Part print with two shaded views. Sizes in mm from the minimum x, y, z corner. A direction names the side the tool comes from. Give positions to 0.01 mm unless a question says otherwise; leave off trailing zeros. Order: outer loops, then holes, each group sorted by start corner. A loop starts at its lowest first (then second) coordinate and runs counter-clockwise, first axis right, second up.
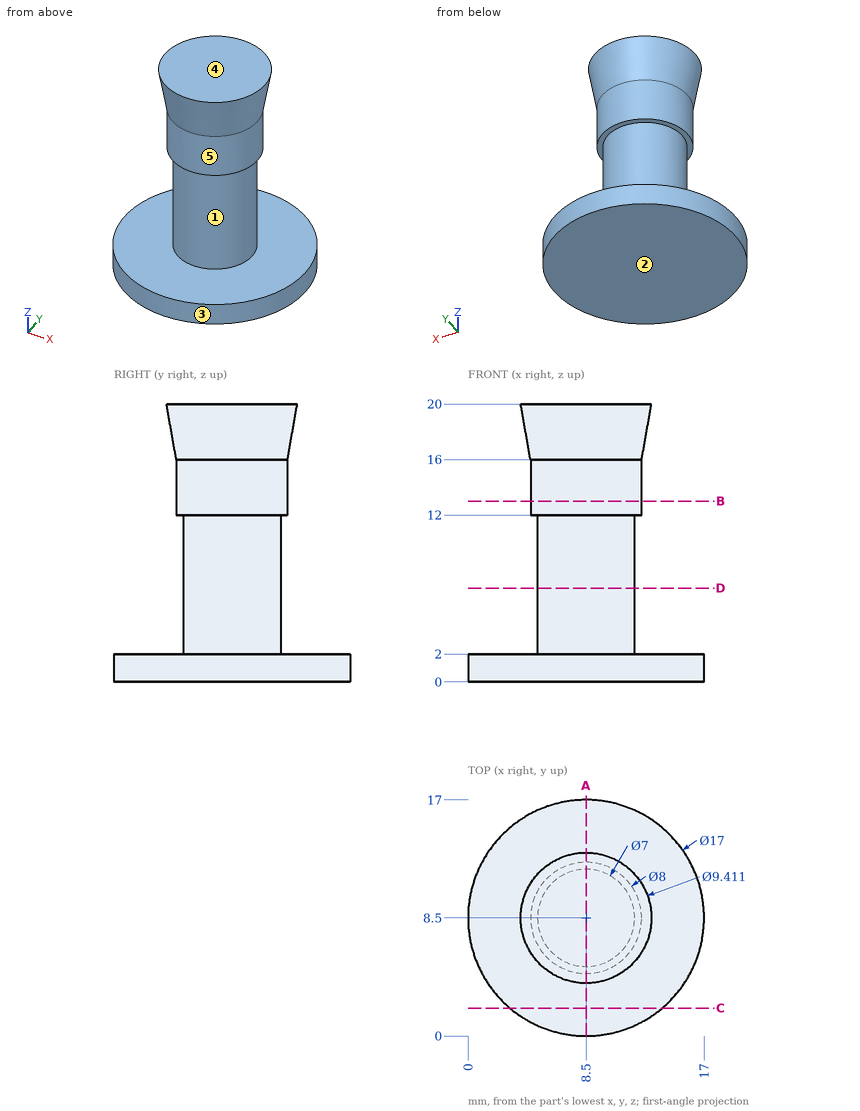
Item 1: Slice it at C-C (y = 2). Give the cut face in (x, z), and give its area (3 significant figures).
Item 2: Two-plate mould, pull along Z, no slides. Class the marked faces 1, 2 and 3: released by +Z, released by -Z, zero draft, split by the parting line, or undercut.
Item 3: Slice it at A-A (x = 8.5). Give the cut face in (y, z) (1 decimal), and give its area (3 significant figures).
Item 4: Tool access for the marked faces 4 and 5: list every direction of +Z, -Z, +X, -X, +Y, -Y with a clear straight run to the whole face (end or side of a thin tool).
Item 5: Drop flat-ended pins along their axis: pin 1 Ø6 at (x, z) = (7, 7.5) entering from -Y; pin 2 Ø8 at (y, z) = (12, 6.5) entering from -X; pin 3 Ø1.5 at (y, z) = (10.5, 14) entering from -X. Give the stop position or say it passes through.
Item 6: Wall check: L1, parallel to Z at x = 15.25, y = 4; L2, parallel to X at y = 7.5, z = 1.75; L3, parallel to X at y = 6, z = 14. Give the ranges that are in metal, low to high.
Item 7: Slice it at D-D (z = 6.75). Give the cut face in (x, y).
Item 8: Slice it at B-B (z = 13). Give the cut face in (x, y).
A:
1. outline: (3.02, 0) - (13.98, 0) - (13.98, 2) - (3.02, 2) - close
1. area: 21.9 mm2
2. face 1: undercut
2. face 2: released by -Z
2. face 3: zero draft
3. outline: (0, 0) - (17, 0) - (17, 2) - (12, 2) - (12, 12) - (12.5, 12) - (12.5, 16) - (13.2, 20) - (3.8, 20) - (4.5, 16) - (4.5, 12) - (5, 12) - (5, 2) - (0, 2) - close
3. area: 171 mm2
4. face 4: +Z, +X, -X, +Y, -Y
4. face 5: none
5. pin 1: stops at y = 5
5. pin 2: stops at x = 5
5. pin 3: stops at x = 4.7
6. L1: z = 0 to 2
6. L2: x = 0.06 to 16.94
6. L3: x = 5.38 to 11.62
7. outline: circle Ø7 at (8.5, 8.5)
8. outline: circle Ø8 at (8.5, 8.5)
